from build123d import *

# Parameters (mm, degrees)
F0_R     = 24.075
F0_W     = 60.15
F0_H     = 4.525
F0_H_2   = 8.95
F0_R_2   = 1.5
F1_DEPTH = 11.75
F2_DEPTH = 5.625
F3_R     = 2.975
F4_DEPTH = 4.63
F5_DEPTH = 8.94
F6_R     = 5


with BuildPart() as f1:
    # F0 (on Top) → F1 (new body)
    with BuildSketch(Plane.XY):
        with BuildLine():
            ThreePointArc((-30.075, 0), (0, -30.075), (30.075, 0))
            ThreePointArc((30.075, 0), (0, 30.075), (-30.075, 0))
        make_face()
        Circle(F0_R, mode=Mode.SUBTRACT)
        with BuildLine():
            Line((30.075, -31), (30.075, 0))
            ThreePointArc((30.075, 0), (0, -30.075), (-30.075, 0))
            Line((-30.075, 0), (-30.075, -31))
            Line((-30.075, -31), (30.075, -31))
        make_face()
        with Locations((0, -33.2625)):
            Rectangle(F0_W, F0_H)
        with Locations((0, -40)):
            Rectangle(F0_W, F0_H_2)
        with Locations((-10.035, -40)):
            Circle(F0_R_2, mode=Mode.SUBTRACT)
        with BuildLine():
            ThreePointArc((10.035, -41.5), (8.535, -40), (10.035, -38.5))
            Line((10.035, -38.5), (12.035, -38.5))
            ThreePointArc((12.035, -38.5), (13.0956601718, -38.9393398282), (13.535, -40))
            ThreePointArc((13.535, -40), (13.0956601718, -41.0606601718), (12.035, -41.5))
            Line((12.035, -41.5), (10.035, -41.5))
        make_face(mode=Mode.SUBTRACT)
        with Locations((0, -46.7375)):
            Rectangle(F0_W, F0_H)
    extrude(amount=F1_DEPTH)

    # F0 (on Top) → F2 (cut)
    with BuildSketch(Plane.XY):
        with Locations((0, -40)):
            Rectangle(F0_W, F0_H_2)
        with Locations((-10.035, -40)):
            Circle(F0_R_2, mode=Mode.SUBTRACT)
        with BuildLine():
            ThreePointArc((10.035, -41.5), (8.535, -40), (10.035, -38.5))
            Line((10.035, -38.5), (12.035, -38.5))
            ThreePointArc((12.035, -38.5), (13.0956601718, -38.9393398282), (13.535, -40))
            ThreePointArc((13.535, -40), (13.0956601718, -41.0606601718), (12.035, -41.5))
            Line((12.035, -41.5), (10.035, -41.5))
        make_face(mode=Mode.SUBTRACT)
    extrude(amount=F2_DEPTH, mode=Mode.SUBTRACT)

    # F3 (on face) → F4 (cut)
    with BuildSketch(Plane.XY.offset(11.75)):
        with Locations((-10.035, -40)):
            Circle(F3_R)
        with BuildLine():
            Line((12.035, -37.025), (10.035, -37.025))
            ThreePointArc((10.035, -37.025), (7.06, -40), (10.035, -42.975))
            Line((10.035, -42.975), (12.035, -42.975))
            ThreePointArc((12.035, -42.975), (15.01, -40), (12.035, -37.025))
        make_face()
        with BuildLine():
            ThreePointArc((10.035, -41.5), (8.535, -40), (10.035, -38.5))
            Line((10.035, -38.5), (12.035, -38.5))
            ThreePointArc((12.035, -38.5), (13.535, -40), (12.035, -41.5))
            Line((12.035, -41.5), (10.035, -41.5))
        make_face(mode=Mode.SUBTRACT)
    extrude(amount=-F4_DEPTH, mode=Mode.SUBTRACT)

    # F0 (on Top) → F5 (cut)
    with BuildSketch(Plane.XY):
        with BuildLine():
            ThreePointArc((-30.075, 0), (0, -30.075), (30.075, 0))
            ThreePointArc((30.075, 0), (0, 30.075), (-30.075, 0))
        make_face()
        Circle(F0_R, mode=Mode.SUBTRACT)
        with BuildLine():
            Line((30.075, -31), (30.075, 0))
            ThreePointArc((30.075, 0), (0, -30.075), (-30.075, 0))
            Line((-30.075, 0), (-30.075, -31))
            Line((-30.075, -31), (30.075, -31))
        make_face()
    extrude(amount=F5_DEPTH, mode=Mode.SUBTRACT)

    # F6
    f6_edges = [f1.edges().sort_by_distance(p)[0] for p in [
        (0, -31, 8.94),
    ]]
    fillet(f6_edges, radius=F6_R)


solid = f1.part
Input: part model. Units: mm. Frame: model coordinates. A direction names the side the tool comes from. Coordinates: 2 decimals unless noted, no trailing zeros. Order: outer loops, then holes, each group sorted by start corner. A loop starts at its lowest first (then second) coordinate and runs counter-clockwise, first axis right, second up. Notation, with made-up numbers: M 79.25,85 L 122.25,85 A35 cw 122.25,122 Z; hole C 45.5,-31 d1. An arc over 180 degrees is marked long. Answer in a Markdown table with one row per item.
(1) Draft query along Y for faces 1 (the flat face through (0, -33, 0)), 2 (the cylindrical face through (15.01, -40.07, 9.47)), 3 (the flat face through (0, -49, 6)), 4 (the flat face through (11, -42.975, 9)). Return one class per face: pulls with the +Y half, pulls with the -Y half, needs draft (parallel to the pull), parting line crosses it, or undercut.
Numbers:
| item | result |
|---|---|
| face 1 | needs draft |
| face 2 | undercut |
| face 3 | pulls with the -Y half |
| face 4 | undercut |
(2) Access query for faces 5 (the flat face through (-30.075, -30, 8)), 6 (the flat face through (0, -47, 0)), 7 (the flat face through (9, -23, 8.94)), 8 (the flat face through (0, -35.525, 3)), 9 (the flat face through (-8.8, -41.3, 7.12)). Directions: +Z, -Z, +X, -X, +Y, -Y. A direction counts if a zero-diameter tool reaches every point of the face in a straight line with its end or side. Return the directions, or none.
Numbers:
| item | result |
|---|---|
| face 5 | +Z, -Z, -X, +Y, -Y |
| face 6 | -Z, +X, -X, +Y, -Y |
| face 7 | -Z, +X, -X, +Y |
| face 8 | -Z, +X, -X |
| face 9 | +Z |
(3) Contact query for flat-ended pins moving along their axis: pin 1 Ø1.7 at (x, z) = (-1.5, 2) entering from +Y; pin 2 Ø5 at (x, y) = (-10.035, -40) entering from +Z; pin 3 Ø0.6 at (x, z) = (11, 9) entering from +Y; pin 4 Ø10 at (x, y) = (-4.5, -39) entering from -Z. Output: stop coordinate, or through.
Numbers:
| item | result |
|---|---|
| pin 1 | stops at y = -31 |
| pin 2 | stops at z = 7.12 |
| pin 3 | stops at y = 28.11 |
| pin 4 | stops at z = 0 |
(4) Section query D-D, the plane z = 10. Output: boundary loops of the cut face in (x, y) (3 decimals), plus the area to 3 significant figures.
Numbers:
| item | result |
|---|---|
| outline | M -30.075,-49 L 30.075,-49 L 30.075,0 A30.075 ccw -30.075,0 Z; hole C 0,0 d48.15; hole C -10.035,-40 d5.95; hole M 10.035,-42.975 L 12.035,-42.975 A2.975 ccw 12.035,-37.025 L 10.035,-37.025 A2.975 ccw Z |
| area | 2,480 mm^2 |
(5) Material intervals for line 1 (X direction, y = -40, z = 6.4) (3 decimals); line 2 (Y direction, x = 9, z = 3.5) (3 decimals); line 3 (Y direction, x = 11.5, z = 11.25) (3 decimals), sorted ascending. Write a range as [from, to].
Numbers:
| item | result |
|---|---|
| line 1 | x = [-30.075, -11.535], [-8.535, 8.535], [13.535, 30.075] |
| line 2 | y = [-49, -44.475], [-35.525, -31] |
| line 3 | y = [-49, -42.975], [-37.025, -21.151], [21.151, 27.789] |
(6) Section query A-A, the plane x = 0. Output: boundary loops of the cut face in (y, z) (3 decimals), plus the area to 3 significant figures.
Numbers:
| item | result |
|---|---|
| outline | M -49,0 L -44.475,0 L -44.475,5.625 L -35.525,5.625 L -35.525,0 L -31,0 L -31,3.94 A5 cw -26,8.94 L -24.075,8.94 L -24.075,11.75 L -49,11.75 Z; M 24.075,8.94 L 30.075,8.94 L 30.075,11.75 L 24.075,11.75 Z |
| area | 203 mm^2 |
(7) Section query C-C, the plane y = 10. Output: boundary loops of the cut face in (x, z).
Numbers:
| item | result |
|---|---|
| outline | M -28.36,8.94 L -21.9,8.94 L -21.9,11.75 L -28.36,11.75 Z; M 21.9,8.94 L 28.36,8.94 L 28.36,11.75 L 21.9,11.75 Z |
(8) Section query B-B, the plane z = 2.25. Output: boundary loops of the cut face in (x, y) (3 decimals).
Numbers:
| item | result |
|---|---|
| outline | M -30.075,-49 L 30.075,-49 L 30.075,-44.475 L -30.075,-44.475 Z; M -30.075,-35.525 L 30.075,-35.525 L 30.075,-31 L -30.075,-31 Z |
